Autodesk Fusion 360 part; units mm, degrees
sketch "Skizze1" plane through (0, 0, 0) normal (0, 0, 1) x (1, 0, 0)
  line L0 (0, 0) -> (111, 0)
  line L1 (111, 0) -> (111, 68)
  line L2 (0, 68) -> (0, 0)
  line L3 (111, 68) -> (0, 68)
  circle A0 centre (79, 60) radius 2
  line L4 (2, 66) -> (109, 66)
  line L5 (109, 66) -> (109, 2)
  line L6 (109, 2) -> (2, 2)
  line L7 (2, 2) -> (2, 66)
  line L8 (2.5, 66) -> (2.5, 65.5)
  line L9 (2.5, 65.5) -> (2, 65.5)
  line L10 (108.5, 2) -> (108.5, 2.5)
  line L11 (108.5, 2.5) -> (109, 2.5)
  line L12 (2.5, 65.5) -> (108.5, 65.5)
  line L13 (108.5, 65.5) -> (108.5, 2.5)
  line L14 (108.5, 2.5) -> (2.5, 2.5)
  line L15 (2.5, 2.5) -> (2.5, 65.5)
  line L16 (5, 9) -> (35, 9)
  line L17 (35, 9) -> (35, 59)
  line L18 (35, 59) -> (5, 59)
  line L19 (5, 59) -> (5, 9)
  line L20 (20, 9) -> (20, 13)
  circle A1 centre (20, 13) radius 1.75
  line L21 (20, 59) -> (20, 55)
  circle A2 centre (20, 55) radius 1.75
  line L22 (75, 15) -> (73, 15)
  line L23 (73, 15) -> (73, 53)
  line L24 (73, 53) -> (75, 53)
  line L25 (75, 53) -> (75, 15)
  line L26 (71, 53) -> (71, 15)
  line L27 (71, 15) -> (69, 15)
  line L28 (69, 53) -> (71, 53)
  line L29 (69, 15) -> (69, 53)
  line L30 (67, 53) -> (67, 15)
  line L31 (67, 15) -> (65, 15)
  line L32 (65, 53) -> (67, 53)
  line L33 (65, 15) -> (65, 53)
  line L34 (63, 53) -> (63, 15)
  line L35 (63, 15) -> (61, 15)
  line L36 (61, 53) -> (63, 53)
  line L37 (61, 15) -> (61, 53)
  line L38 (59, 53) -> (59, 15)
  line L39 (59, 15) -> (57, 15)
  line L40 (57, 53) -> (59, 53)
  line L41 (57, 15) -> (57, 53)
  line L42 (55, 53) -> (55, 15)
  line L43 (55, 15) -> (53, 15)
  line L44 (53, 53) -> (55, 53)
  line L45 (53, 15) -> (53, 53)
  line L46 (51, 53) -> (51, 15)
  line L47 (51, 15) -> (49, 15)
  line L48 (49, 53) -> (51, 53)
  line L49 (49, 15) -> (49, 53)
  line L50 (47, 53) -> (47, 15)
  line L51 (47, 15) -> (45, 15)
  line L52 (45, 53) -> (47, 53)
  line L53 (45, 15) -> (45, 53)
  line L54 (0, 60) -> (77, 60)
  line L55 (79, 60) -> (79, 66)
  dimension "d9" = 111
  dimension "d10" = 68
  dimension "d13" = 4
  dimension "d30" = 0.5
  dimension "d31" = 0.5
  dimension "d32" = 30
  dimension "d33" = 50
  dimension "d34" = 3.5
  dimension "d35" = 4
  dimension "d36" = 3.5
  dimension "d72" = 2
  dimension "d73" = 38
  dimension "d76" = -28
  dimension "d77" = 0
  dimension "d110" = 77
  dimension "d111" = 6
extrude "Extrusion5" add sketch "Skizze1" along normal blind 2 contours L7 L9 L15 L54 | L6 L7 L10 L14 L15 L54 | L0 L1 L2 L3 | L4 L7 L8 L9 | A0 L12 L13 L14 L15 L54 L55 | A0 L12 L15 L54 L55 | L5 L6 L10 L11 | L4 L8 L12 L55 | L4 L5 L11 L12 L13 L55 | L16 L17 L18 L19
sketch "Skizze3" plane through (0, 53, 0) normal (0, -1, 0) x (1, 0, 0)
  line L0 (73, 0) -> (75, 0)
  line L1 (75, 0) -> (75, 2)
  line L2 (75, 2) -> (73, 2)
  line L3 (73, 2) -> (73, 0)
  line L4 (73, 2) -> (75, 0)
  line L5 (73, 0) -> (71, 2)
  line L6 (71, 2) -> (73, 2)
  line L7 (75, 0) -> (73, 0)
  line L8 (73, 0) -> (71.183, 0)
  line L9 (71.183, 0) -> (71, 2)
  line L10 (71.183, 0) -> (71, 2)
  line L11 (75, 0) -> (75, 2)
  line L12 (73, 2) -> (75, 2)
  line L13 (69, 0) -> (67, 2)
  line L14 (71, 0) -> (71, 2)
  line L15 (69, 2) -> (69, 0)
  line L16 (71, 2) -> (69, 2)
  line L17 (69, 2) -> (71, 2)
  line L18 (71, 0) -> (71, 2)
  line L19 (69, 0) -> (67.183, 0)
  line L20 (69, 2) -> (71, 0)
  line L21 (69, 0) -> (71, 0)
  line L22 (67.183, 0) -> (67, 2)
  line L23 (67, 2) -> (69, 2)
  line L24 (67.183, 0) -> (67, 2)
  line L25 (71, 0) -> (69, 0)
  line L26 (65, 0) -> (63, 2)
  line L27 (67, 0) -> (67, 2)
  line L28 (65, 2) -> (65, 0)
  line L29 (67, 2) -> (65, 2)
  line L30 (65, 2) -> (67, 2)
  line L31 (67, 0) -> (67, 2)
  line L32 (65, 0) -> (63.183, 0)
  line L33 (65, 2) -> (67, 0)
  line L34 (65, 0) -> (67, 0)
  line L35 (63.183, 0) -> (63, 2)
  line L36 (63, 2) -> (65, 2)
  line L37 (63.183, 0) -> (63, 2)
  line L38 (67, 0) -> (65, 0)
  line L39 (61, 0) -> (59, 2)
  line L40 (63, 0) -> (63, 2)
  line L41 (61, 2) -> (61, 0)
  line L42 (63, 2) -> (61, 2)
  line L43 (61, 2) -> (63, 2)
  line L44 (63, 0) -> (63, 2)
  line L45 (61, 0) -> (59.183, 0)
  line L46 (61, 2) -> (63, 0)
  line L47 (61, 0) -> (63, 0)
  line L48 (59.183, 0) -> (59, 2)
  line L49 (59, 2) -> (61, 2)
  line L50 (59.183, 0) -> (59, 2)
  line L51 (63, 0) -> (61, 0)
  line L52 (57, 0) -> (55, 2)
  line L53 (59, 0) -> (59, 2)
  line L54 (57, 2) -> (57, 0)
  line L55 (59, 2) -> (57, 2)
  line L56 (57, 2) -> (59, 2)
  line L57 (59, 0) -> (59, 2)
  line L58 (57, 0) -> (55.183, 0)
  line L59 (57, 2) -> (59, 0)
  line L60 (57, 0) -> (59, 0)
  line L61 (55.183, 0) -> (55, 2)
  line L62 (55, 2) -> (57, 2)
  line L63 (55.183, 0) -> (55, 2)
  line L64 (59, 0) -> (57, 0)
  line L65 (53, 0) -> (51, 2)
  line L66 (55, 0) -> (55, 2)
  line L67 (53, 2) -> (53, 0)
  line L68 (55, 2) -> (53, 2)
  line L69 (53, 2) -> (55, 2)
  line L70 (55, 0) -> (55, 2)
  line L71 (53, 0) -> (51.183, 0)
  line L72 (53, 2) -> (55, 0)
  line L73 (53, 0) -> (55, 0)
  line L74 (51.183, 0) -> (51, 2)
  line L75 (51, 2) -> (53, 2)
  line L76 (51.183, 0) -> (51, 2)
  line L77 (55, 0) -> (53, 0)
  line L78 (49, 0) -> (47, 2)
  line L79 (51, 0) -> (51, 2)
  line L80 (49, 2) -> (49, 0)
  line L81 (51, 2) -> (49, 2)
  line L82 (49, 2) -> (51, 2)
  line L83 (51, 0) -> (51, 2)
  line L84 (49, 0) -> (47.183, 0)
  line L85 (49, 2) -> (51, 0)
  line L86 (49, 0) -> (51, 0)
  line L87 (47.183, 0) -> (47, 2)
  line L88 (47, 2) -> (49, 2)
  line L89 (47.183, 0) -> (47, 2)
  line L90 (51, 0) -> (49, 0)
  line L91 (45, 0) -> (43, 2)
  line L92 (47, 0) -> (47, 2)
  line L93 (45, 2) -> (45, 0)
  line L94 (47, 2) -> (45, 2)
  line L95 (45, 2) -> (47, 2)
  line L96 (47, 0) -> (47, 2)
  line L97 (45, 0) -> (43.183, 0)
  line L98 (45, 2) -> (47, 0)
  line L99 (45, 0) -> (47, 0)
  line L100 (43.183, 0) -> (43, 2)
  line L101 (43, 2) -> (45, 2)
  line L102 (43.183, 0) -> (43, 2)
  line L103 (47, 0) -> (45, 0)
  dimension "d80" = -28
  dimension "d81" = 0
extrude "Extrusion8" add sketch "Skizze3" along normal blind 38 contours L92 L94 L95 L96 L98 | L79 L81 L82 L83 L85 | L66 L68 L69 L70 L72 | L53 L55 L56 L57 L59 | L40 L42 L43 L44 L46 | L27 L29 L30 L31 L33 | L14 L16 L17 L18 L20 | L1 L2 L4 L11 L12
extrude "Extrusion9" cut sketch "Skizze3" along normal blind 38 contours L0 L3 L4 L7 | L3 L5 L6 | L15 L20 L21 L25 | L13 L15 L23 | L28 L33 L34 L38 | L26 L28 L36 | L41 L46 L47 L51 | L39 L41 L49 | L54 L59 L60 L64 | L52 L54 L62 | L67 L72 L73 L77 | L65 L67 L75 | L80 L85 L86 L90 | L78 L80 L88 | L93 L98 L99 L103 | L91 L93 L101
sketch "Skizze5" plane through (0, 0, 0) normal (0, 0, 1) x (1, 0, 0)
  line L0 (111, 68) -> (0, 68)
  line L1 (2, 66) -> (109, 66)
  line L2 (108.5, 2) -> (108.5, 2.5)
  line L3 (108.5, 2.5) -> (2.5, 2.5)
  line L4 (0, 0) -> (111, 0)
  line L5 (109, 66) -> (109, 2)
  line L6 (108.5, 2.5) -> (109, 2.5)
  line L7 (2.5, 65.5) -> (108.5, 65.5)
  line L8 (111, 0) -> (111, 68)
  line L9 (2.5, 66) -> (2.5, 65.5)
  line L10 (108.5, 65.5) -> (108.5, 2.5)
  line L11 (109, 2) -> (2, 2)
  line L12 (2, 2) -> (2, 66)
  line L13 (2.5, 65.5) -> (2, 65.5)
  line L14 (0, 68) -> (0, 0)
  line L15 (2.5, 2.5) -> (2.5, 65.5)
  line L16 (108.5, 65.5) -> (104.5, 65.5)
  line L17 (104.5, 65.5) -> (104.5, 61.5)
  line L18 (2.5, 2.5) -> (2.5, 6.5)
  line L19 (2.5, 6.5) -> (6.5, 6.5)
  line L20 (104.5, 61.5) -> (6.5, 61.5)
  line L21 (6.5, 61.5) -> (6.5, 6.5)
  line L22 (6.5, 6.5) -> (104.5, 6.5)
  line L23 (104.5, 6.5) -> (104.5, 61.5)
  circle A0 centre (79, 60) radius 2
  circle A1 centre (79, 60) radius 3
  line L24 (82.5, 61.5) -> (75, 61.5)
  dimension "d138" = 111
  dimension "d139" = 68
  dimension "d141" = 0.5
  dimension "d142" = 0.5
  dimension "d152" = 4
  dimension "d153" = 4
  dimension "d154" = 4
  dimension "d155" = 4
  dimension "d156" = 6
extrude "Extrusion15" add sketch "Skizze5" against normal blind 1.5 contours L7 L15 L17 L19 L20 L21 A1 L24 | L3 L7 L10 L15 L16 L17 L18 L19 L22 L23
sketch "Skizze2" plane through (0, 0, 0) normal (0, -1, 0) x (1, 0, 0)
  line L0 (0, 0) -> (111, 0)
  line L1 (111, 2) -> (0, 2)
  line L2 (0, 2) -> (0, 0)
  circle A0 centre (7, -17) radius 1.75
  line L3 (8.75, -17) -> (10.25, -17)
  line L4 (7.0687, -18.7487) -> (7.0687, -20.2487)
  line L5 (5.25, -17) -> (3.75, -17)
  line L6 (3.75, -17) -> (3.75, -20.25)
  line L7 (3.75, -20.25) -> (7.0687, -20.2487)
  line L8 (7.0687, -20.2487) -> (10.25, -20.25)
  line L9 (10.25, -20.25) -> (10.25, -17)
  line L10 (3.75, -17) -> (3.75, 0)
  line L11 (10.25, -17) -> (10.25, 0)
  line L12 (0, 0) -> (7, 0)
  line L13 (7, 0) -> (7, -17)
  line L14 (55.5, 0) -> (55.5, -30)
  line L15 (0, 0) -> (111, 0)
  line L16 (111, 2) -> (0, 2)
  line L17 (0, 2) -> (0, 0)
  line L18 (5.4123, -14.25) -> (3.8246, -17)
  line L19 (3.8246, -17) -> (5.4123, -19.75)
  line L20 (5.4123, -19.75) -> (8.5877, -19.75)
  line L21 (8.5877, -19.75) -> (10.14, -16.9898)
  line L22 (10.14, -16.9898) -> (8.5877, -14.25)
  line L23 (8.5877, -14.25) -> (5.4123, -14.25)
  line L24 (3, -13.5) -> (11, -13.5)
  line L25 (11, -13.5) -> (11, -20.5)
  line L26 (11, -20.5) -> (3, -20.5)
  line L27 (3, -20.5) -> (3, -13.5)
  line L28 (105.5877, -14.25) -> (107.1754, -17)
  line L29 (100.75, -20.25) -> (100.75, -17)
  line L30 (100, -20.5) -> (108, -20.5)
  line L31 (100.86, -16.9898) -> (102.4123, -14.25)
  line L32 (102.4123, -19.75) -> (100.86, -16.9898)
  line L33 (102.25, -17) -> (100.75, -17)
  line L34 (107.25, -20.25) -> (103.9313, -20.2487)
  line L35 (104, 0) -> (104, -17)
  line L36 (108, -20.5) -> (108, -13.5)
  line L37 (103.9313, -20.2487) -> (100.75, -20.25)
  line L38 (102.4123, -14.25) -> (105.5877, -14.25)
  line L39 (107.1754, -17) -> (105.5877, -19.75)
  circle A1 centre (104, -17) radius 1.75
  line L40 (105.5877, -19.75) -> (102.4123, -19.75)
  line L41 (107.25, -17) -> (107.25, 0)
  line L42 (103.9313, -18.7487) -> (103.9313, -20.2487)
  line L43 (105.75, -17) -> (107.25, -17)
  line L44 (100.75, -17) -> (100.75, 0)
  line L45 (108, -13.5) -> (100, -13.5)
  line L46 (107.25, -17) -> (107.25, -20.25)
  line L47 (100, -13.5) -> (100, -20.5)
  dimension "d46" = 3.5
  dimension "d56" = 1.5
  dimension "d57" = 1.5
  dimension "d58" = 1.5
  dimension "d59" = 7
  dimension "d96" = 8
  dimension "d97" = 7
extrude "Extrusion16" add sketch "Skizze2" against normal blind 6 from surface at -2.5 contours L0 L15 L35 L44 L45 | L0 L10 L12 L13 L15 L24 | L0 L11 L13 L15 L24 | L5 L10 L13 L18 L23 L24 | L6 L7 L8 L9 L10 L11 L24 L25 L26 L27 | L3 L11 L13 L21 L22 L23 L24 | L4 L5 L6 L7 L19 L20 | A0 L3 L13 L21 L22 L23 | A0 L5 L13 L18 L23 | A0 L4 L5 L19 L20 | L3 L4 L8 L9 L20 L21 | L0 L15 L35 L41 L45 | L31 L32 L33 L35 L38 L44 L45 | L29 L30 L34 L36 L37 L41 L44 L45 L46 L47 | A0 L3 L4 L20 L21 | L28 L35 L38 L41 L43 L45 | L29 L32 L33 L37 L40 L42 | L28 L35 L38 A1 L43 | L31 L32 L33 L35 L38 A1 | L32 L33 A1 L40 L42 | L34 L39 L40 L42 L43 L46 | L39 A1 L40 L42 L43
extrude "Extrusion17" cut sketch "Skizze2" along normal blind 2.75 from surface at -8.5 contours A0 L3 L13 L21 L22 L23 | A0 L5 L13 L18 L23 | A0 L4 L5 L19 L20 | A0 L3 L4 L20 L21 | L28 L35 L38 A1 L43 | L31 L32 L33 L35 L38 A1 | L32 L33 A1 L40 L42 | L39 A1 L40 L42 L43
extrude "Extrusion18" add sketch "Skizze2" along normal blind 6 from surface at -65.5 contours L0 L15 L35 L44 L45 | L0 L15 L35 L41 L45 | L31 L32 L33 L35 L38 L44 L45 | L29 L30 L34 L36 L37 L41 L44 L45 L46 L47 | L28 L35 L38 L41 L43 L45 | L29 L32 L33 L37 L40 L42 | L28 L35 L38 A1 L43 | L31 L32 L33 L35 L38 A1 | L32 L33 A1 L40 L42 | L34 L39 L40 L42 L43 L46 | L39 A1 L40 L42 L43
extrude "Extrusion19" cut sketch "Skizze2" against normal blind 2.75 from surface at -59.5 contours L28 L35 L38 A1 L43 | L31 L32 L33 L35 L38 A1 | L32 L33 A1 L40 L42 | L39 A1 L40 L42 L43
sketch "Skizze6" plane through (0, 0, 0) normal (0, 0, -1) x (1, 0, 0)
  line L0 (100.75, -61.5) -> (100.75, -59.5)
  line L1 (100.75, -59.5) -> (104.5, -59.5)
  line L2 (104.5, -59.5) -> (104.5, -8.5)
  line L3 (104.5, -8.5) -> (100.75, -8.5)
  line L4 (100.75, -8.5) -> (100.75, -6.5)
  line L5 (100.75, -6.5) -> (10.25, -6.5)
  line L6 (10.25, -6.5) -> (10.25, -8.5)
  line L7 (10.25, -8.5) -> (6.5, -8.5)
  line L8 (6.5, -8.5) -> (6.5, -61.5)
  line L9 (6.5, -61.5) -> (76.4019, -61.5)
  arc A0 (76.4019, -61.5) -> (81.5981, -61.5) centre (79, -60) ccw
  line L10 (81.5981, -61.5) -> (100.75, -61.5)
  line L11 (61, -15) -> (63, -15)
  line L12 (63, -15) -> (63, -53)
  line L13 (63, -53) -> (61, -53)
  line L14 (61, -53) -> (61, -15)
  line L15 (75, -53) -> (73, -53)
  line L16 (73, -53) -> (73, -15)
  line L17 (73, -15) -> (75, -15)
  line L18 (75, -15) -> (75, -53)
  line L19 (49, -15) -> (51, -15)
  line L20 (51, -15) -> (51, -53)
  line L21 (51, -53) -> (49, -53)
  line L22 (49, -53) -> (49, -15)
  line L23 (69, -15) -> (71, -15)
  line L24 (71, -15) -> (71, -53)
  line L25 (71, -53) -> (69, -53)
  line L26 (69, -53) -> (69, -15)
  line L27 (53, -15) -> (55, -15)
  line L28 (55, -15) -> (55, -53)
  line L29 (55, -53) -> (53, -53)
  line L30 (53, -53) -> (53, -15)
  circle A1 centre (79, -60) radius 2
  line L31 (57, -15) -> (59, -15)
  line L32 (59, -15) -> (59, -53)
  line L33 (59, -53) -> (57, -53)
  line L34 (57, -53) -> (57, -15)
  circle A2 centre (20, -13) radius 1.75
  line L35 (65, -15) -> (67, -15)
  line L36 (67, -15) -> (67, -53)
  line L37 (67, -53) -> (65, -53)
  line L38 (65, -53) -> (65, -15)
  circle A3 centre (20, -55) radius 1.75
  line L39 (45, -15) -> (47, -15)
  line L40 (47, -15) -> (47, -53)
  line L41 (47, -53) -> (45, -53)
  line L42 (45, -53) -> (45, -15)
Geometry: final body of the model. Coordinates: model frame, mm. A direction names the side the tool comes from. Coordinates: 2 decimals unless noted, no trailing zeros. Write each loop counter-clockwise with the first axis right and the second up, starting at its lowest first coordinate (ties: lowest second). Pieces come first, ordered by that corner, then holes. Notation, with made-up numbers: (87, 85.5) - (130, 85.5) arc R13 ccw to (130, 102.5) - close; hole circle Ø11 at (-33.75, 5). An arc over 180 degrees is marked (long way). Return JSON: item names as keys, results as strings.
Item 1: Section query A-A (x = 79). Output: boundary loops of the cut face in (y, z), and give its area (3 significant figures).
Completed:
{"outline": "(0, 0) - (2.5, 0) - (2.5, -1.5) - (6.5, -1.5) - (6.5, 0) - (58, 0) - (58, 2) - (0, 2) - close; (62, 0) - (63, 0) - (63, -1.5) - (65.5, -1.5) - (65.5, 0) - (68, 0) - (68, 2) - (62, 2) - close", "area": "138 mm2"}
Item 2: Section query C-C (y = 13). Output: boundary loops of the cut face in (x, z), and give its area (3 significant figures).
Completed:
{"outline": "(0, 0) - (2.5, 0) - (2.5, -1.5) - (6.5, -1.5) - (6.5, 0) - (18.25, 0) - (18.25, 2) - (0, 2) - close; (21.75, 0) - (104.5, 0) - (104.5, -1.5) - (108.5, -1.5) - (108.5, 0) - (111, 0) - (111, 2) - (21.75, 2) - close", "area": "227 mm2"}
Item 3: Section query B-B (z = -4). Output: boundary loops of the cut face in (x, y), and give its area (3 significant figures).
Completed:
{"outline": "(3.75, 2.5) - (10.25, 2.5) - (10.25, 8.5) - (3.75, 8.5) - close; (100.75, 2.5) - (107.25, 2.5) - (107.25, 8.5) - (100.75, 8.5) - close; (100.75, 59.5) - (107.25, 59.5) - (107.25, 65.5) - (100.75, 65.5) - close", "area": "117 mm2"}
Item 4: Line query: L1, parallel to X at y = 4.9, z = -17; L2, parallel to Y at x = 20, z = 0.65; L3, parallel to Y at x = 79, z = 1.5. Output: solid intervals per line, ascending.
Completed:
{"L1": "x = 3 to 5.25, 8.75 to 11, 100 to 102.25, 105.75 to 108", "L2": "y = 0 to 11.25, 14.75 to 53.25, 56.75 to 68", "L3": "y = 0 to 58, 62 to 68"}
Item 5: Pull-direction query (X, two-part tool) for faces 5 (the face through (56, 68, 1)), 6 (the face through (0, 34, 1)), 7 (the face through (72, 34, 1)); classes: +X half, -X half, draft (parallel to the pull), parting line (faces both ways), or undercut.
Completed:
{"face 5": "draft", "face 6": "-X half", "face 7": "undercut"}
Item 6: Section query D-D (x = 20). Output: boundary loops of the cut face in (y, z), and give its area (3 significant figures).
Completed:
{"outline": "(0, 0) - (2.5, 0) - (2.5, -1.5) - (6.5, -1.5) - (6.5, 0) - (11.25, 0) - (11.25, 2) - (0, 2) - close; (14.75, 0) - (53.25, 0) - (53.25, 2) - (14.75, 2) - close; (56.75, 0) - (61.5, 0) - (61.5, -1.5) - (65.5, -1.5) - (65.5, 0) - (68, 0) - (68, 2) - (56.75, 2) - close", "area": "134 mm2"}
Item 7: Pin query (flat end, axial travel): pin 1 Ø12 at (x, z) = (14, -9) entering from +Y; pin 2 Ø1.8 at (y, z) = (61, -8) entering from +X; pin 3 Ø6.5 at (y, z) = (61.5, -18) entering from -X. Return the tip coordinate at first contact, or that it passes through.
Completed:
{"pin 1": "stops at y = 8.5", "pin 2": "stops at x = 107.25", "pin 3": "stops at x = 100"}
Item 8: Reachability of faces 1 (the face through (51, 1, 0)), 2 (the face through (104, 61, -14.25)), 3 (the face through (103.772, 4.102, -15.265)), 4 (the face through (79, 65.5, -1)) from +Z, -Z, +X, -X, +Y, -Y: full face, straight path, thin tool, end or side. Return the list, or none.
Completed:
{"face 1": "-Z", "face 2": "none", "face 3": "+Y, -Y", "face 4": "-Z, +X, -X, +Y"}
